from build123d import *

# Parameters (mm, degrees)
GRUNDK_RPER_DEPTH = 4


with BuildPart() as part:
    # Skizze1 → Grundkörper (new body)
    with BuildSketch(Plane.XY):
        with BuildLine():
            Line((-8, 4), (0, 6))
            Line((0, 6), (8, 4))
            ThreePointArc((8, 4), (12, 0), (8, -4))
            Line((8, -4), (0, -6))
            Line((0, -6), (-8, -4))
            ThreePointArc((-8, -4), (-12, 0), (-8, 4))
        make_face()
        with BuildLine():
            ThreePointArc((1.198457832, 2.75021796), (1.104373658, 2.789329458), (1.009015584, 2.825223452))
            ThreePointArc((1.009015584, 2.825223452), (0.81445938, 3.172109853), (0.476854681, 2.961859148))
            ThreePointArc((0.476854681, 2.961859148), (0.375999701, 2.976344104), (0.274711003, 2.987395833))
            ThreePointArc((0.274711003, 2.987395833), (0, 3.275), (-0.274711003, 2.987395833))
            ThreePointArc((-0.274711003, 2.987395833), (-0.375999701, 2.976344104), (-0.476854681, 2.961859148))
            ThreePointArc((-0.476854681, 2.961859148), (-0.81445938, 3.172109853), (-1.009015584, 2.825223452))
            ThreePointArc((-1.009015584, 2.825223452), (-1.104373658, 2.789329458), (-1.198457832, 2.75021796))
            ThreePointArc((-1.198457832, 2.75021796), (-1.577743283, 2.869904377), (-1.679920005, 2.48553189))
            ThreePointArc((-1.679920005, 2.48553189), (-1.763355757, 2.427050983), (-1.844757469, 2.365770462))
            ThreePointArc((-1.844757469, 2.365770462), (-2.241891772, 2.387372255), (-2.245268875, 1.989665218))
            ThreePointArc((-2.245268875, 1.989665218), (-2.311539728, 1.912271969), (-2.375144211, 1.832672906))
            ThreePointArc((-2.375144211, 1.832672906), (-2.765173956, 1.754832754), (-2.669539243, 1.368780564))
            ThreePointArc((-2.669539243, 1.368780564), (-2.714481157, 1.277337875), (-2.756291906, 1.184421771))
            ThreePointArc((-2.756291906, 1.184421771), (-3.114710091, 1.012030657), (-2.926072642, 0.661890392))
            ThreePointArc((-2.926072642, 0.661890392), (-2.946861752, 0.562143944), (-2.964251643, 0.46174906))
            ThreePointArc((-2.964251643, 0.46174906), (-3.268537536, 0.205638951), (-2.998750137, -0.086588787))
            ThreePointArc((-2.998750137, -0.086588787), (-2.994080185, -0.188371559), (-2.985956549, -0.289937043))
            ThreePointArc((-2.985956549, -0.289937043), (-3.216990746, -0.613673805), (-2.883005131, -0.829627274))
            ThreePointArc((-2.883005131, -0.829627274), (-2.853169549, -0.927050983), (-2.820042823, -1.023405335))
            ThreePointArc((-2.820042823, -1.023405335), (-2.963308597, -1.39442718), (-2.58611031, -1.520537228))
            ThreePointArc((-2.58611031, -1.520537228), (-2.532983777, -1.607480385), (-2.476935434, -1.692569306))
            ThreePointArc((-2.476935434, -1.692569306), (-2.52343087, -2.087563566), (-2.126720668, -2.115906237))
            ThreePointArc((-2.126720668, -2.115906237), (-2.053641318, -2.186905882), (-1.978193083, -2.255382922))
            ThreePointArc((-1.978193083, -2.255382922), (-1.924996701, -2.649530657), (-1.533701344, -2.578325074))
            ThreePointArc((-1.533701344, -2.578325074), (-1.445261022, -2.62892004), (-1.355153586, -2.676482535))
            ThreePointArc((-1.355153586, -2.676482535), (-1.20560791, -3.045017991), (-0.844313924, -2.878738265))
            ThreePointArc((-0.844313924, -2.878738265), (-0.746069661, -2.905749483), (-0.646964804, -2.929408907))
            ThreePointArc((-0.646964804, -2.929408907), (-0.41046634, -3.249175647), (-0.101875155, -2.998269743))
            ThreePointArc((-0.101875155, -2.998269743), (0, -3), (0.101875155, -2.998269743))
            ThreePointArc((0.101875155, -2.998269743), (0.41046634, -3.249175647), (0.646964804, -2.929408907))
            ThreePointArc((0.646964804, -2.929408907), (0.746069661, -2.905749483), (0.844313924, -2.878738265))
            ThreePointArc((0.844313924, -2.878738265), (1.20560791, -3.045017991), (1.355153586, -2.676482535))
            ThreePointArc((1.355153586, -2.676482535), (1.445261022, -2.62892004), (1.533701344, -2.578325074))
            ThreePointArc((1.533701344, -2.578325074), (1.924996701, -2.649530657), (1.978193083, -2.255382922))
            ThreePointArc((1.978193083, -2.255382922), (2.053641318, -2.186905882), (2.126720668, -2.115906237))
            ThreePointArc((2.126720668, -2.115906237), (2.52343087, -2.087563566), (2.476935434, -1.692569306))
            ThreePointArc((2.476935434, -1.692569306), (2.532983777, -1.607480385), (2.58611031, -1.520537228))
            ThreePointArc((2.58611031, -1.520537228), (2.963308597, -1.39442718), (2.820042823, -1.023405335))
            ThreePointArc((2.820042823, -1.023405335), (2.853169549, -0.927050983), (2.883005131, -0.829627274))
            ThreePointArc((2.883005131, -0.829627274), (3.216990746, -0.613673805), (2.985956549, -0.289937043))
            ThreePointArc((2.985956549, -0.289937043), (2.994080185, -0.188371559), (2.998750137, -0.086588787))
            ThreePointArc((2.998750137, -0.086588787), (3.268537536, 0.205638951), (2.964251643, 0.46174906))
            ThreePointArc((2.964251643, 0.46174906), (2.946861752, 0.562143944), (2.926072642, 0.661890392))
            ThreePointArc((2.926072642, 0.661890392), (3.114710091, 1.012030657), (2.756291906, 1.184421771))
            ThreePointArc((2.756291906, 1.184421771), (2.714481157, 1.277337875), (2.669539243, 1.368780564))
            ThreePointArc((2.669539243, 1.368780564), (2.765173956, 1.754832754), (2.375144211, 1.832672906))
            ThreePointArc((2.375144211, 1.832672906), (2.311539728, 1.912271969), (2.245268875, 1.989665218))
            ThreePointArc((2.245268875, 1.989665218), (2.241891772, 2.387372255), (1.844757469, 2.365770462))
            ThreePointArc((1.844757469, 2.365770462), (1.763355757, 2.427050983), (1.679920005, 2.48553189))
            ThreePointArc((1.679920005, 2.48553189), (1.577743283, 2.869904377), (1.198457832, 2.75021796))
        make_face(mode=Mode.SUBTRACT)
    extrude(amount=GRUNDK_RPER_DEPTH)


solid = part.part
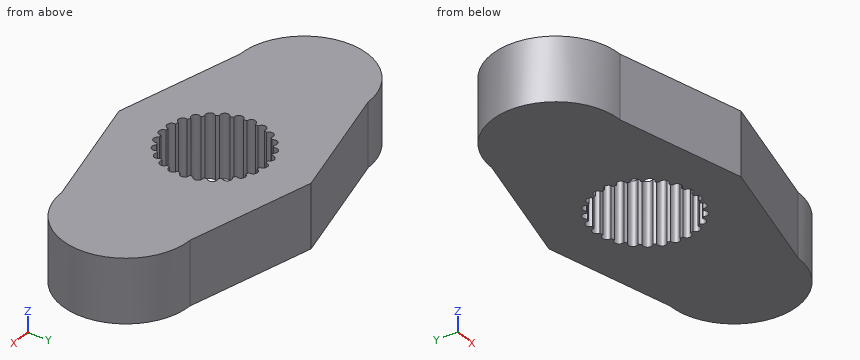
Source: CAD feature listing. Evaluate the final solid. Frame: model axes, mm. Round coordinates to 2 decimals unless told otherwise and drop trailing zeros. Write each loop counter-clockwise with the first axis right and the second up, starting at its lowest first coordinate (ties: lowest second). Pieces come first, ordered by that corner, then holes. Notation, with made-up numbers: (13, 47.25) - (43, 47.25) arc R28 cw to (43, 76.25) - close; hole circle Ø9 at (-6.5, 76). An arc over 180 degrees is marked (long way). Use CSV: the item, a comma, the result in double quotes. Start each with the question number.
(1) Cut plane B-B, the plane x = 5.5. Return loops of the section in (y, z) (3 decimals).
(2) First-contact query: pin 1 Ø2 at (y, z) = (-3.5, 1.5) entering from -X. Flat tip, straight axial feed; report the tip coordinate or a pass-through.
(3) Material intervals for probe 1 along X at (y, z) = (-0.75, 2.7); probe 2 along X at (y, z) = (0, 3.35); probe 3 along Y at (x, z) = (-0.75, 1.75), sorted ascending. Write a range as [from, to].
(4) Cut plane A-A, the plane y = 4.5. Return loops of the section in (x, z), and give its area (3 significant figures).
Geometry says:
1,outline,"(-4.625, 0) - (4.625, 0) - (4.625, 4) - (-4.625, 4) - close"
2,pin 1,"x = -11.12"
3,probe 1,"[-11.93, -3.15], [3.15, 11.93]"
3,probe 2,"[-12, -3.19], [3.19, 12]"
3,probe 3,"[-5.81, -2.9], [3.18, 5.81]"
4,outline,"(-6, 0) - (6, 0) - (6, 4) - (-6, 4) - close"
4,area,"48.0 mm²"
